from build123d import *

# Parameters (mm, degrees)
SKETCH1_R           = 1.5
SKETCH1_W           = 25
SKETCH1_H           = 35
BOSS_EXTRUDE1_DEPTH = 3.125
FILLET2_R           = 15
FILLET3_R           = 30
FILLET4_R           = 30
FILLET5_R           = 80
FILLET6_R           = 30
FILLET7_R           = 5
FILLET1_R           = 10
FILLET8_R           = 5


with BuildPart() as part:
    # Sketch1 → Boss-Extrude1 (new body)
    with BuildSketch(Plane(origin=(0, 0, 0), x_dir=(0, 0, -1), z_dir=(1, 0, 0))):
        Polygon((-143.20422433, -1.13137085), (-143.20422433, -26.13137085), (-64.062088707, -26.13137085), (-52.930717857, -15), (19.6, -15), (19.6, 49.830569927), (-31.940768363, 49.830569927), (-82.90270914, -1.13137085), (-98.20422433, -1.13137085), (-98.20422433, 43.86862915), (-143.20422433, 43.86862915), align=None)
        with Locations((-46.799347007, 3.010764774)):
            Circle(SKETCH1_R, mode=Mode.SUBTRACT)
        with Locations((-14.979541854, 34.830569927)):
            Circle(SKETCH1_R, mode=Mode.SUBTRACT)
        with Locations((-73.810826048, -0.524769132)):
            Circle(SKETCH1_R, mode=Mode.SUBTRACT)
        with Locations((-73.20422433, -16.13137085)):
            Circle(SKETCH1_R, mode=Mode.SUBTRACT)
        with Locations((-133.20422433, -16.13137085)):
            Circle(SKETCH1_R, mode=Mode.SUBTRACT)
        with Locations((-138.20422433, 38.86862915)):
            Circle(SKETCH1_R, mode=Mode.SUBTRACT)
        with Locations((-103.20422433, 38.86862915)):
            Circle(SKETCH1_R, mode=Mode.SUBTRACT)
        with BuildLine():
            Line((-4.6, 0.75), (-1.854049622, 0.75))
            ThreePointArc((-1.854049622, 0.75), (0, 2), (1.854049622, 0.75))
            Line((1.854049622, 0.75), (4.6, 0.75))
            ThreePointArc((4.6, 0.75), (5.35, 0), (4.6, -0.75))
            Line((4.6, -0.75), (1.854049622, -0.75))
            ThreePointArc((1.854049622, -0.75), (0, -2), (-1.854049622, -0.75))
            Line((-1.854049622, -0.75), (-4.6, -0.75))
            ThreePointArc((-4.6, -0.75), (-5.35, 0), (-4.6, 0.75))
        make_face(mode=Mode.SUBTRACT)
        Polygon((-35.667976157, 0), (-10.83740623, 24.830569927), (-0.4, 24.830569927), (-0.4, 13.742135624), (-14.142135624, 0), align=None, mode=Mode.SUBTRACT)
        with Locations((-120.70422433, 16.36862915)):
            Rectangle(SKETCH1_W, SKETCH1_H, mode=Mode.SUBTRACT)
    extrude(amount=BOSS_EXTRUDE1_DEPTH)

    # Fillet2
    fillet2_edges = [part.edges().sort_by_distance(p)[0] for p in [
        (1.5625, -15, 52.930717857),
        (1.5625, -26.13137085, 64.062088707),
    ]]
    fillet(fillet2_edges, radius=FILLET2_R)

    # Fillet3
    fillet3_edges = [part.edges().sort_by_distance(p)[0] for p in [
        (1.5625, -15, -19.6),
    ]]
    fillet(fillet3_edges, radius=FILLET3_R)

    # Fillet4
    fillet4_edges = [part.edges().sort_by_distance(p)[0] for p in [
        (1.5625, 49.830569927, 31.940768363),
    ]]
    fillet(fillet4_edges, radius=FILLET4_R)

    # Fillet5
    # the kernel refuses this fillet: 80 mm, written as the material it adds along each edge
    with BuildSketch(Plane(origin=(0, -1.13137085, 82.90270914), x_dir=(0, 0.7071067811865434, -0.7071067811865517), z_dir=(1, 0, 0))) as fillet5_piece_1:
        with BuildLine():
            CenterArc((29.356066225, 80), FILLET5_R, 239.854448647, 30.145551353)
            Line((-10.819805153, 10.819805153), (-11.623322581, 9.436201256))
            ThreePointArc((-11.623322581, 9.436201256), (-6.541273427, 4.278531727), (-1.13137085, -1.13137085))
            Line((-1.13137085, -1.13137085), (0, -1.6))
            Line((0, -1.6), (29.356066225, -1.6))
            Line((29.356066225, -1.6), (29.356066225, 0))
        make_face()
    extrude(amount=3.125)

    # Fillet6
    fillet6_edges = [part.edges().sort_by_distance(p)[0] for p in [
        (1.5625, 49.830569927, -19.6),
    ]]
    fillet(fillet6_edges, radius=FILLET6_R)

    # Fillet7
    fillet7_edges = [part.edges().sort_by_distance(p)[0] for p in [
        (1.5625, 13.742135624, 0.4),
        (1.5625, 24.830569927, 0.4),
        (1.5625, 24.830569927, 10.83740623),
        (1.5625, 0, 35.667976157),
        (1.5625, 0, 14.142135624),
    ]]
    fillet(fillet7_edges, radius=FILLET7_R)

    # Fillet1
    fillet1_edges = [part.edges().sort_by_distance(p)[0] for p in [
        (1.5625, -26.13137085, 143.20422433),
    ]]
    fillet(fillet1_edges, radius=FILLET1_R)

    # Fillet8
    fillet8_edges = [part.edges().sort_by_distance(p)[0] for p in [
        (1.5625, 43.86862915, 143.20422433),
        (1.5625, 43.86862915, 98.20422433),
        (1.5625, -1.13137085, 98.20422433),
        (1.5625, 33.86862915, 133.20422433),
        (1.5625, -1.13137085, 133.20422433),
        (1.5625, -1.13137085, 108.20422433),
        (1.5625, 33.86862915, 108.20422433),
    ]]
    fillet(fillet8_edges, radius=FILLET8_R)


solid = part.part
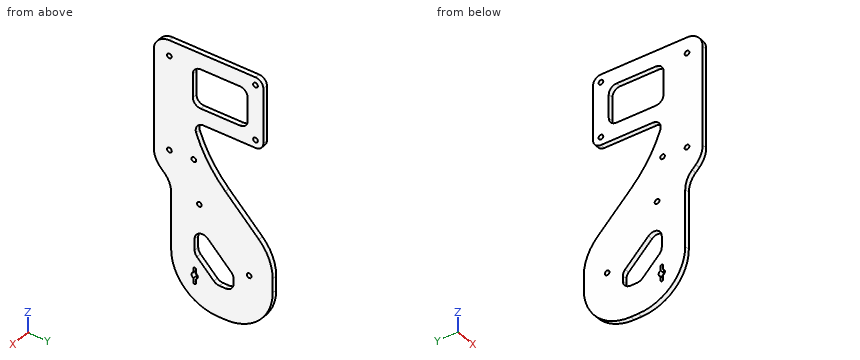
CAD build for the part. Positions are in the model's coordinates, mm. Coordinates: 2 decimals unless noted, no trailing zeros. Order: outer loops, then holes, each group sorted by start corner. A loop starts at its lowest first (then second) coordinate and runs counter-clockwise, first axis right, second up.
Item 1: Drill centre lines: L1, parallel to Z at x = 1.5, y = 29.5; L2, parallel to Y at x = 2.35, z = 74; L3, parallel to Z at x = 1.4, y = 21. Where is each one in solid material? Low to high.
Check sheet entries:
L1: z = -18 to 52.27, 98.2 to 108.24, 133.16 to 143.2
L2: y = -26.13 to -17.4, -14.86 to -2.01, 0.96 to 9.86
L3: z = -19.58 to 0.54, 14.67 to 60.77, 98.2 to 108.2, 133.2 to 143.2
Item 2: Band-saw the part on A-A on z = 120. List the corners of the cut face in (x, y) (3 decimals), plus the area to 3 significant figures.
Check sheet entries:
outline: (0, -26.131) - (3.125, -26.131) - (3.125, -1.131) - (0, -1.131) - close; (0, 33.869) - (3.125, 33.869) - (3.125, 43.869) - (0, 43.869) - close
area: 109 mm2
Item 3: Band-saw the part on C-C on z = 37. List the corners of the cut face in (x, y) (3 decimals), plus the area to 3 significant figures.
Check sheet entries:
outline: (0, -15) - (3.125, -15) - (3.125, 44.208) - (0, 44.208) - close
area: 185 mm2
Item 4: Pin check, flat tips, straight feed: pin 1 Ø0.9 at (x, z) = (1, 6.5) entering from -Y; pin 2 Ø0.9 at (x, y) = (2, 11) entering from -Z; pin 3 Ø0.8 at (x, z) = (1, 2.5) entering from -Y. Stop position of each tip, or through.
Check sheet entries:
pin 1: stops at y = -14.8
pin 2: stops at z = -19.39
pin 3: stops at y = -14.05
Item 5: Band-saw the part on B-B on x = 1.05. Give the number of separate pieces and of enclosed holes in the cut face, plus the area to 3 significant figures.
Check sheet entries:
separate pieces: 1
enclosed holes: 10
area: 7,450 mm2
